Here's the drawing with two shaded views (mm, measured from the low corner). I have some questions. Coordinates: 2 decimals unless noted, no trailing zeros. Write each loop counter-clockwise with the first axis right and the second up, starting at its lowest first coordinate (ties: lowest second). Pieces come first, ordered by that corner, then holes.
Item 1: I'm going to push a flat-ended pin straight in: pin 1 Ø0.6 at (x, z) = (19.5, 0.5) entering from -Y. Where does the tip first touch, or does it pass through?
Item 2: We'd pull the mould along Y, two halves only. Please class the marked faces 1, 2 and 3: +Y half, -Y half, draft (parallel to the pull), parting line (faces both ways), or undercut.
Item 3: If I drill on line 1 (X direction, y = 3, z = 9.25); line 2 (Y direction, x = 20.5, z = 5.5) (3 decimals); line 3 (Y direction, x = 20.5, z = 1.75) (3 decimals), over which ranges is the centre line in solid material (lowest first)?
Item 4: If we section it at A-A (x = 9.5): Please give me the cut outline in (y, z) (3 decimals), then the cut area to 4 significant figures.
Item 5: If we section it at B-B (z = 5.1): Please give me the cut outline in (x, y) (3 decimals), then the cut area to 3 significant figures.
Item 6: If we section it at C-C (y = 4.75): Please give me the cut outline in (x, z), then the cut area to 3 significant figures.
Item 7: If we section it at D-D (x = 17): Please give me the cut outline in (y, z).
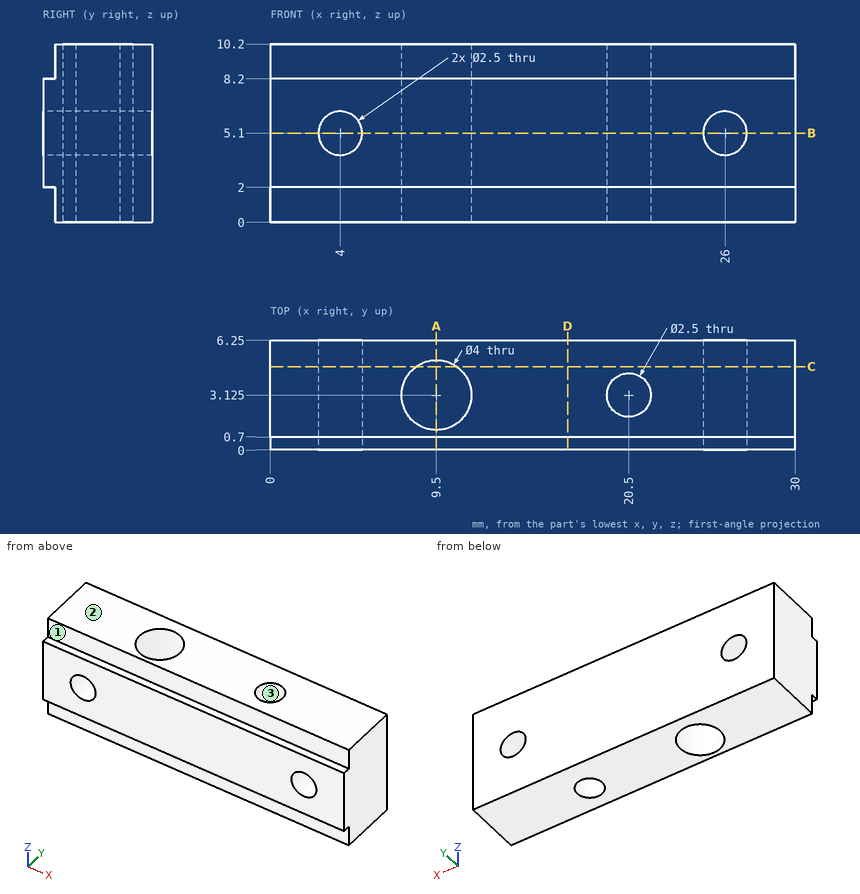
Answer list:
1. pin 1: stops at y = 0.7
2. face 1: -Y half
2. face 2: draft
2. face 3: undercut
3. line 1: x = 0 to 7.5, 11.5 to 19.26, 21.74 to 30
3. line 2: y = 0 to 1.875, 4.375 to 6.25
3. line 3: y = 0.7 to 1.875, 4.375 to 6.25
4. outline: (0, 2) - (0.7, 2) - (0.7, 0) - (1.125, 0) - (1.125, 10.2) - (0.7, 10.2) - (0.7, 8.2) - (0, 8.2) - close; (5.125, 0) - (6.25, 0) - (6.25, 10.2) - (5.125, 10.2) - close
4. area: 20.15 mm2
5. outline: (0, 0) - (2.75, 0) - (2.75, 6.25) - (0, 6.25) - close; (5.25, 0) - (24.75, 0) - (24.75, 6.25) - (5.25, 6.25) - close; (27.25, 0) - (30, 0) - (30, 6.25) - (27.25, 6.25) - close; hole circle Ø4 at (9.5, 3.125); hole circle Ø2.5 at (20.5, 3.125)
5. area: 139 mm2
6. outline: (0, 0) - (8.33, 0) - (8.33, 10.2) - (0, 10.2) - close; (10.67, 0) - (30, 0) - (30, 10.2) - (10.67, 10.2) - close; hole circle Ø2.5 at (4, 5.1); hole circle Ø2.5 at (26, 5.1)
6. area: 272 mm2
7. outline: (0, 2) - (0.7, 2) - (0.7, 0) - (6.25, 0) - (6.25, 10.2) - (0.7, 10.2) - (0.7, 8.2) - (0, 8.2) - close
